Autodesk Inventor part; units mm, degrees
ref_plane "YZ Plane" through (0, 0, 0) normal (1, 0, 0) x (0, 1, 0)
ref_plane "XZ Plane" through (0, 0, 0) normal (0, 1, 0) x (-1, 0, 0)
ref_plane "XY Plane" through (0, 0, 0) normal (0, 0, 1) x (1, 0, 0)
sketch "Sketch1" plane through (0, 0, 0) normal (0, 0, 1) x (1, 0, 0)
  circle A0 centre (0, 0) radius 24.5
  circle A1 centre (0, 0) radius 30
  dimension "d0" = 49
  dimension "d1" = 60
extrude "Extrusion1" add sketch "Sketch1" against normal blind 1.1
sketch "Sketch2" plane through (0, 0, 0) normal (0, 0, 1) x (1, 0, 0)
  line L0 (0, 0) -> (0, 30) construction
  circle A0 centre (0, 0) radius 30 construction
  line L1 (-1.73, 27.25) -> (2.3469, 27.25) construction
  line L2 (2.3469, 27.25) -> (2.3469, 25.3632) construction
  line L3 (2.3469, 25.3632) -> (-1.73, 25.3632) construction
  line L4 (-1.73, 25.3632) -> (-1.73, 27.25) construction
  line L5 (-1.4916, 25.85) -> (2.1084, 25.85)
  line L6 (2.1084, 25.85) -> (2.1084, 28.65)
  line L7 (2.1084, 28.65) -> (-1.4916, 28.65)
  line L8 (-1.4916, 28.65) -> (-1.4916, 25.85)
  line L9 (-1.4916, 25.85) -> (2.1084, 28.65) construction
  line L10 (2.1084, 25.85) -> (-1.4916, 28.65) construction
  point P0 (0.3084, 27.25)
  dimension "d4" = 27.25
  dimension "d5" = 2.8
  dimension "d6" = 3.6
extrude "Extrusion2" add sketch "Sketch2" along normal blind 1.7
pattern_circular "Circular Pattern1" count 15 over 360 about axis through (0, 0, -10) along (0, 0, 1) of "Extrusion2"
properties part number "Light Ring"
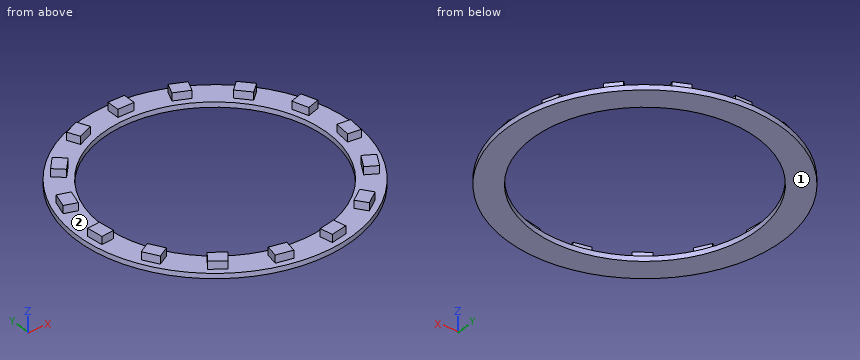
Can you work these out from the model? Positions are in its coordinate system, mm. Face numbers are marked on the shaded views. Round coordinates to 2 decimals unless told otherwise and drop trailing zeros. Loops run counter-clockwise (first coordinate to the right, second up) from the corner with the lowest first, then second, coordinate; pieces in that order, holes last.
Item 1: If we mould it in two halves opening along X, with no side actions, what happens to the marked faces 1 and 2? For each: +X half, -X half, draft (parallel to the pull), parting line (faces both ways), or undercut.
Item 2: Please list where these lines run through material, in increasing order: L1, parallel to Y at x = 0, z = -0.4; L2, parallel to Z at x = -1, y = -27; L3, parallel to X at y = -20.5, z = -0.8.
Item 3: Suppose I cut it at B-B, the plane z = 0.7. State how many separate pieces and enclosed holes the cut face has, then the cut area to 3 significant figures.
Item 4: Suppose I cut it at C-C, the plane y = 14.5. Write out the boundary of the cut face in (x, z), then the cut area to 3 significant figures.
Item 5: Will these pins go through, and if not, where does the flat tip stop? pin 1 Ø1.5 at (x, z) = (4, 0) entering from +Y; pin 2 Ø1 at (y, z) = (20.5, 1) entering from -X; pin 3 Ø0.8 at (y, z) = (28, 1) entering from -X.
Item 6: Suppose I cut it at A-A, the plane x = 0. Write out the boundary of the cut face in (y, z), then the cut area to 3 significant figures.
Item 7: Suppose I cut it at D-D, the plane x = 19. Write out the boundary of the cut face in (y, z).
Reported:
1. face 1: draft
1. face 2: undercut
2. L1: y = -30 to -24.5, 24.5 to 30
2. L2: z = -1.1 to 0
2. L3: x = -21.9 to -13.42, 13.42 to 21.9
3. separate pieces: 15
3. enclosed holes: 0
3. area: 151 mm2
4. outline: (-26.26, -1.1) - (-19.75, -1.1) - (-19.75, 0) - (-26.26, 0) - close; (19.75, -1.1) - (26.26, -1.1) - (26.26, 0) - (19.75, 0) - close
4. area: 14.3 mm2
5. pin 1: stops at y = 29.82
5. pin 2: stops at x = -20.54
5. pin 3: stops at x = -1.49
6. outline: (-30, -1.1) - (-24.5, -1.1) - (-24.5, 0) - (-30, 0) - close; (24.5, -1.1) - (30, -1.1) - (30, 0) - (28.65, 0) - (28.65, 1.7) - (25.85, 1.7) - (25.85, 0) - (24.5, 0) - close
6. area: 16.9 mm2
7. outline: (-23.22, -1.1) - (-15.47, -1.1) - (-15.47, 0) - (-23.22, 0) - close; (15.47, -1.1) - (23.22, -1.1) - (23.22, 0) - (19.11, 0) - (19.11, 1.7) - (17.53, 1.7) - (17.53, 0) - (15.47, 0) - close
